Input: part model. Units: mm. Frame: model coordinates. Give positions to 0.01 mm unless a question says otherwise; leave off trailing zeros. Loops run counter-clockwise (first coordinate to the right, second up) from the corner with the lowest first, then second, coordinate; pieces in that order, holes last.
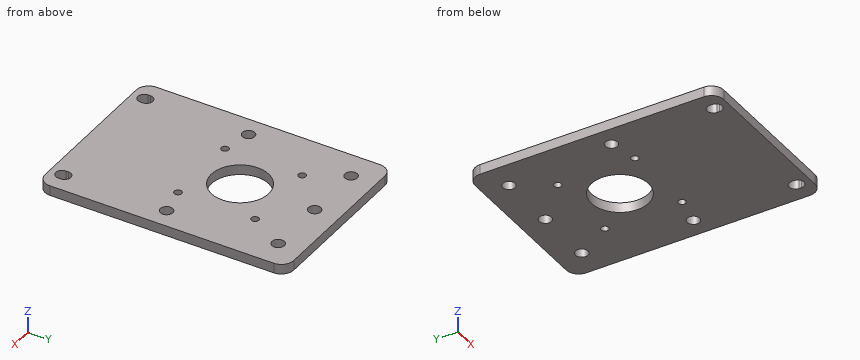
from build123d import *

# Parameters (mm, degrees)
SKETCH4_W           = 70
SKETCH4_H           = 100
SKETCH4_R           = 2.5
BOSS_EXTRUDE2_DEPTH = 4
SKETCH5_R           = 11.5
SKETCH5_R_2         = 1.5
CUT_EXTRUDE2_DEPTH  = 5
SKETCH6_R           = 2.5
CUT_EXTRUDE3_DEPTH  = 5
FILLET1_R           = 5


with BuildPart() as part:
    # Sketch4 → Boss-Extrude2 (new body)
    with BuildSketch(Plane.XY):
        Rectangle(SKETCH4_W, SKETCH4_H)
        with Locations((-27, -3)):
            Circle(SKETCH4_R, mode=Mode.SUBTRACT)
        with Locations((27, -3)):
            Circle(SKETCH4_R, mode=Mode.SUBTRACT)
        with BuildLine():
            Line((-24.5, -44), (-24.5, -45))
            ThreePointArc((-24.5, -45), (-27, -47.5), (-29.5, -45))
            Line((-29.5, -45), (-29.5, -44))
            ThreePointArc((-29.5, -44), (-27, -41.5), (-24.5, -44))
        make_face(mode=Mode.SUBTRACT)
        with BuildLine():
            Line((24.5, -44), (24.5, -45))
            ThreePointArc((24.5, -45), (27, -47.5), (29.5, -45))
            Line((29.5, -45), (29.5, -44))
            ThreePointArc((29.5, -44), (27, -41.5), (24.5, -44))
        make_face(mode=Mode.SUBTRACT)
    extrude(amount=BOSS_EXTRUDE2_DEPTH)

    # Sketch5 → Cut-Extrude2 (cut, through all)
    with BuildSketch(Plane.XY.offset(4)):
        with Locations((0, 10.076696831)):
            Circle(SKETCH5_R)
        with Locations((-15.5, 25.576696831)):
            Circle(SKETCH5_R_2)
        with Locations((15.5, 25.576696831)):
            Circle(SKETCH5_R_2)
        with Locations((15.5, -5.423303169)):
            Circle(SKETCH5_R_2)
        with Locations((-15.5, -5.423303169)):
            Circle(SKETCH5_R_2)
    extrude(amount=-CUT_EXTRUDE2_DEPTH, mode=Mode.SUBTRACT)

    # Sketch6 → Cut-Extrude3 (cut, through all)
    with BuildSketch(Plane.XY.offset(4)):
        with Locations((24, 40.076696831)):
            Circle(SKETCH6_R)
        with Locations((-24, 40.076696831)):
            Circle(SKETCH6_R)
        with Locations((0, 40.076696831)):
            Circle(SKETCH6_R)
    extrude(amount=-CUT_EXTRUDE3_DEPTH, mode=Mode.SUBTRACT)

    # Fillet1
    fillet1_edges = [part.edges().sort_by_distance(p)[0] for p in [
        (35, -50, 2),
        (-35, -50, 2),
        (-35, 50, 2),
        (35, 50, 2),
    ]]
    fillet(fillet1_edges, radius=FILLET1_R)


solid = part.part
(1) Pin query (flat end, axial travel): pin 1 Ø6 at (x, y) = (27, -3) entering from -Z. Return the tip coordinate at first contact, or that it passes through.
Values follow:
pin 1: stops at z = 0
(2) Cut plane C-C (x = -6). Return the cut outline in (y, z).
Values follow:
outline: (-50, 0) - (0.27, 0) - (0.27, 4) - (-50, 4) - close; (19.89, 0) - (50, 0) - (50, 4) - (19.89, 4) - close
(3) Cut plane A-A (x = -15.5). Return the cut outline in (y, z), and give its area (3 significant figures).
Values follow:
outline: (-50, 0) - (-6.92, 0) - (-6.92, 4) - (-50, 4) - close; (-3.92, 0) - (24.08, 0) - (24.08, 4) - (-3.92, 4) - close; (27.08, 0) - (50, 0) - (50, 4) - (27.08, 4) - close
area: 376 mm2
(4) Cut plane B-B (z = 1.05). Count the separate pieces of the cut face and the enclosed holes in it, and give its area (3 significant figures).
Values follow:
separate pieces: 1
enclosed holes: 12
area: 6,390 mm2
(5) Ray query, probe 1 along Y at (x, z) = (-15.5, 2.25); probe 2 along Y at (x, z) = (27, 2.1); probe 3 along X at (y, z) = (38, 0.9). Return the intervals inside material, ascending.
Values follow:
probe 1: y = -50 to -6.92, -3.92 to 24.08, 27.08 to 50
probe 2: y = -50 to -47.5, -41.5 to -5.5, -0.5 to 50
probe 3: x = -35 to -25.39, -22.61 to -1.39, 1.39 to 22.61, 25.39 to 35
(6) Cut plane D-D (y = 16). Return the cut outline in (x, z), and give its area (3 significant figures).
Values follow:
outline: (-35, 0) - (-9.86, 0) - (-9.86, 4) - (-35, 4) - close; (9.86, 0) - (35, 0) - (35, 4) - (9.86, 4) - close
area: 201 mm2
